from build123d import *

# Parameters (mm, degrees)
SKETCH_W        = 100
SKETCH_H        = 65
PAD_DEPTH       = 20
SKETCH001_W     = 25
SKETCH001_H     = 35
PAD001_DEPTH    = 60
SKETCH002_W     = 18.940022
SKETCH002_H     = 50
PAD002_DEPTH    = 80
PAD003_DEPTH    = 25
POCKET_DEPTH    = 75
POCKET001_DEPTH = 65.001


with BuildPart() as part:
    # Sketch → Pad (new body)
    with BuildSketch(Plane.XY):
        Rectangle(SKETCH_W, SKETCH_H)
    extrude(amount=PAD_DEPTH)

    # Sketch001 → Pad001 (new body)
    with BuildSketch(Plane.XY.offset(20)):
        with Locations((-37.5, -15)):
            Rectangle(SKETCH001_W, SKETCH001_H)
    extrude(amount=PAD001_DEPTH)

    # Sketch002 → Pad002 (new body)
    with BuildSketch(Plane.XY.offset(80)):
        with Locations((-54.470011, 7.5)):
            Rectangle(SKETCH002_W, SKETCH002_H)
    extrude(amount=-PAD002_DEPTH)

    # Sketch003 → Pad003 (new body)
    with BuildSketch(Plane.XY.offset(20)):
        Polygon((-45, 32.5), (50, 32.5), (50, -32.5), (-25, -32.5), (-25, 2.5), (-45, 2.5), align=None)
    extrude(amount=PAD003_DEPTH)

    # Sketch004 → Pocket (cut)
    with BuildSketch(Plane.YZ.offset(50)):
        Polygon((-32.5, 45), (2.5, 45), (-32.5, 20), align=None)
    extrude(amount=-POCKET_DEPTH, mode=Mode.SUBTRACT)

    # Sketch005 → Pocket001 (cut, through all)
    with BuildSketch(Plane(origin=(0, 32.5, 0), x_dir=(-1, 0, 0), z_dir=(0, 1, 0))):
        Polygon((-50, 20), (0, 45), (-50, 45), align=None)
    extrude(amount=-POCKET001_DEPTH, mode=Mode.SUBTRACT)


solid = part.part
Could you check a few things on this model? Use its own coordinates, in mm. A direction names the side the tool comes from. Give positions to 0.01 mm unless a question says otherwise; leave off trailing zeros. Order: outer loops, then holes, each group sorted by start corner. A loop starts at its lowest first (then second) coordinate and runs counter-clockwise, first axis right, second up.
1. Suppose I cut it at A-A (z = 64.5). List the corners of the cut face in (x, y) for me, plus the area to 3 significant figures.
2. For faces 1 (the flat face through (-50, -25, 39)), 2 (the flat face through (4.69, -18.64, 29.9)), 3 (the flat face through (25.35, 7.677, 32.325)), 4 (the flat face through (-45, 17, 63)), which set-ups out of +Z, -Z, +X, -X, +Y, -Y let a thin tool reach every point of the face, with its end or its side?
3. Will these pins go through, and if not, where does the flat tip stop? P1, Ø7, axis at x = -56.5, z = 36, coming from the -Y side; P2, Ø4, axis at y = 23, z = 22.5, coming from the +X side; P3, Ø10, axis at x = -39, z = 57.5, coming from the +Y side.
4. Suppose I cut it at C-C (x = 15). List the corners of the cut face in (y, z) for me.
5. I need wall thicknesses on L1, parallel to X at y = -13.5, z = 71.5; L2, parallel to Y at x = -55, z = 10.5; L3, parallel to X at y = -21.5, z = 45. Which ranges of each line are inside material? Lowest first, please.
6. Suppose I cut it at B-B (y = 10.5). List the corners of the cut face in (x, z) for me.
7. Suppose I cut it at D-D (x = 33). List the corners of the cut face in (y, z) for me, plus the area to 3 significant figures.
Solved:
1. outline: (-63.94, -17.5) - (-50, -17.5) - (-50, -32.5) - (-25, -32.5) - (-25, 2.5) - (-45, 2.5) - (-45, 32.5) - (-63.94, 32.5) - close
1. area: 1,720 mm2
2. face 1: +Z, -Z, -X, -Y
2. face 2: +Z, +X, -Y
2. face 3: +Z, +X, +Y, -Y
2. face 4: +Z, +X, +Y
3. P1: stops at y = -17.5
3. P2: stops at x = 49
3. P3: stops at y = 2.5
4. outline: (-32.5, 0) - (32.5, 0) - (32.5, 37.5) - (-8, 37.5) - (-32.5, 20) - close
5. L1: x = -63.94 to -25
5. L2: y = -17.5 to 32.5
5. L3: x = -50 to -25
6. outline: (-63.94, 0) - (50, 0) - (50, 20) - (0, 45) - (-45, 45) - (-45, 80) - (-63.94, 80) - close
7. outline: (-32.5, 0) - (32.5, 0) - (32.5, 28.5) - (-20.6, 28.5) - (-32.5, 20) - close
7. area: 1,800 mm2
